Read the model definition and answer for the solid it produces. Units are mm, in the model's axes. Give positions to 0.01 mm unless a question says otherwise; leave off trailing zeros. Loops run counter-clockwise (first coordinate to the right, second up) from the corner with the lowest first, then second, coordinate; pieces in that order, holes last. Notation, with made-up numbers: (-35, 78.25) - (-16, 78.25) arc R26 cw to (-16, 105.25) - close; hole circle Ø1 at (26.25, 85.5). An arc over 180 degrees is marked (long way). Write each question's results on one line, items separated by ' | '. Start each with the question number.
Q1. The part is cut by section B-B, the plane y = -8. Write down the section's boundary in (x, z).
Q2. The part is cut by section A-A, the plane x = 1. Write down the section's boundary in (y, z), plus the area to 3 significant figures.
Q3. Given pin 1 (1 mm diameter, centred on x = -27.5, z = 1.5, fed in from +Y); pin 2 (2 mm diameter, centred on y = -69, z = 2.5, fed in from -X); pin 3 (3 mm diameter, centred on x = -99.53, z = 3, fed in from -Y), each flat-ended and moving along its own axis, determine where each tip first touches the part or whether it passes through.
Q4. Find the intervals of material crossed by line 1 (Y direction, x = -26, z = 3.1); line 2 (Y direction, x = -8, z = 1.5); line 3 (Y direction, x = -81, z = 0.5), in increasing order. Write a range as from..to.
```python
from build123d import *

# Parameters (mm, degrees)
SKETCH_2_R          = 4
EXTRUDE_1_DEPTH     = 6
SKETCH_3_R          = 1.25
CUT_EXTRUDE_1_DEPTH = 5
CUT_EXTRUDE_START   = -5
SKETCH_4_R          = 1.25
CUT_EXTRUDE_2_DEPTH = 5
SKETCH_5_R          = 1.25
CUT_EXTRUDE_3_DEPTH = 5
SKETCH_6_R          = 1.25
CUT_EXTRUDE_4_DEPTH = 5
SKETCH_8_R          = 1.25
CUT_EXTRUDE_5_DEPTH = 5
SKETCH_9_R          = 1.25
CUT_EXTRUDE_6_DEPTH = 5
FILLET_2_R          = 3


with BuildPart() as part:
    # 스케치2 → 보스-돌출1 (new body)
    with BuildSketch(Plane.XY):
        with BuildLine():
            Line((-102.525284978, -57.601148056), (-102.525284978, -32.601148056))
            Line((-102.525284978, -32.601148056), (-80.525284978, -32.601148056))
            ThreePointArc((-80.525284978, -32.601148056), (-73.11411316, -27.970582536), (-68.384824454, -20.622015799))
            Line((-68.384824454, -20.622015799), (-68.384824454, 23.377984201))
            Line((-68.384824454, 23.377984201), (-43.384824454, 23.377984201))
            Line((-43.384824454, 23.377984201), (-43.545565494, 1.378571429))
            ThreePointArc((-43.545565494, 1.378571429), (-38.886846868, -5.94242943), (-31.565846009, -10.601148056))
            Line((-31.565846009, -10.601148056), (12.434153991, -10.601148056))
            Line((12.434153991, -10.601148056), (12.434153991, -35.601148056))
            Line((12.434153991, -35.601148056), (-9.565846009, -35.601148056))
            ThreePointArc((-9.565846009, -35.601148056), (-16.886846868, -40.259866682), (-21.545565494, -47.580867541))
            Line((-21.545565494, -47.580867541), (-21.545565494, -91.580867541))
            Line((-21.545565494, -91.580867541), (-46.545565494, -91.580867541))
            Line((-46.545565494, -91.580867541), (-46.545565494, -69.580867541))
            ThreePointArc((-46.545565494, -69.580867541), (-51.20428412, -62.259866682), (-58.525284978, -57.601148056))
            Line((-58.525284978, -57.601148056), (-102.525284978, -57.601148056))
        make_face()
        with Locations((-43.384824454, -32.601148056)):
            Circle(SKETCH_2_R, mode=Mode.SUBTRACT)
    extrude(amount=EXTRUDE_1_DEPTH)

    # 스케치3 → 컷-돌출1 (cut)
    with BuildSketch(Plane(origin=(0, -57.601148056, 0), x_dir=(-1, 0, 0), z_dir=(0, -1, 0))):
        with Locations(Location((99.525284978, -3, 0), (0, 0, 90))):
            Circle(SKETCH_3_R)
    extrude(amount=-CUT_EXTRUDE_1_DEPTH, mode=Mode.SUBTRACT)

    # 스케치4 → 컷-돌출2 (cut)
    with BuildSketch(Plane(origin=(0, -32.601148056, 0), x_dir=(1, 0, 0), z_dir=(0, 1, 0)).offset(CUT_EXTRUDE_START)):
        with Locations(Location((-99.525284978, -3, 0), (0, 0, 90))):
            Circle(SKETCH_4_R)
    extrude(amount=CUT_EXTRUDE_2_DEPTH, mode=Mode.SUBTRACT)

    # 스케치5 → 컷-돌출3 (cut)
    with BuildSketch(Plane(origin=(-21.545565494, 0, 0), x_dir=(0, 0, -1), z_dir=(1, 0, 0))):
        with Locations(Location((-3.087647422, -88.347802665, 0), (0, 0, 90))):
            Circle(SKETCH_5_R)
    extrude(amount=-CUT_EXTRUDE_3_DEPTH, mode=Mode.SUBTRACT)

    # 스케치6 → 컷-돌출4 (cut)
    with BuildSketch(Plane.ZY.offset(46.545565494).offset(CUT_EXTRUDE_START)):
        with Locations(Location((3.087647422, -88.347802665, 0), (0, 0, 90))):
            Circle(SKETCH_6_R)
    extrude(amount=CUT_EXTRUDE_4_DEPTH, mode=Mode.SUBTRACT)

    # 스케치8 → 컷-돌출5 (cut)
    with BuildSketch(Plane(origin=(0, -10.601148056, 0), x_dir=(1, 0, 0), z_dir=(0, 1, 0))):
        with Locations(Location((9.434153991, -3, 0), (0, 0, 180))):
            Circle(SKETCH_8_R)
    extrude(amount=-CUT_EXTRUDE_5_DEPTH, mode=Mode.SUBTRACT)

    # 스케치9 → 컷-돌출6 (cut)
    with BuildSketch(Plane(origin=(0, -35.601148056, 0), x_dir=(-1, 0, 0), z_dir=(0, -1, 0)).offset(CUT_EXTRUDE_START)):
        with Locations((-9.434153991, -3)):
            Circle(SKETCH_9_R)
    extrude(amount=CUT_EXTRUDE_6_DEPTH, mode=Mode.SUBTRACT)

    # 필렛2
    fillet_2_edges = [part.edges().sort_by_distance(p)[0] for p in [
        (12.434153991, -23.101148056, 0),
        (12.434153991, -23.101148056, 6),
        (-34.045565494, -91.580867541, 0),
        (-34.045565494, -91.580867541, 6),
        (-102.525284978, -45.101148056, 0),
        (-102.525284978, -45.101148056, 6),
    ]]
    fillet(fillet_2_edges, radius=FILLET_2_R - 0.0001)  # a hair under: the kernel refuses the full size


solid = part.part
```
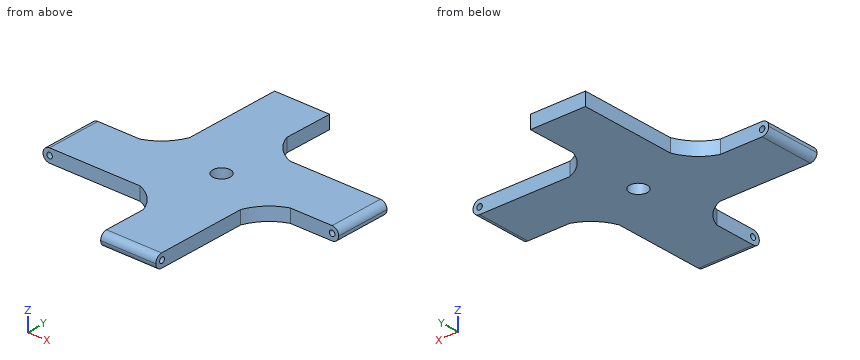
Check sheet entries:
1) outline: (-68.38, 0) - (-36.47, 0) - (-36.47, 6) - (-68.38, 6) - close
2) outline: (-35.6, 0) - (-10.6, 0) - (-10.6, 6) - (-35.6, 6) - close | area: 150 mm^2
3) pin 1: stops at y = -10.6 | pin 2: stops at x = -47.2 | pin 3: stops at y = -57.6
4) line 1: y = -91.58..-89.6, -87.1..-10.6 | line 2: y = -35.6..-10.6 | line 3: y = -57.6..-32.6
